For this review, take the finished solid that the model builds, in its own axes (mm). Face numbers are marked on the shaded views. Coordinates: 2 decimals unless noted, no trailing zeros. Write each loop counter-clockwise with the first axis right and the second up, starting at its lowest first coordinate (ties: lowest second). Pieces come first, ordered by that corner, then holes. Notation, with made-up numbers: (-20, 86) - (-8, 86) arc R23 ccw to (-8, 125) - close; hole circle Ø1 at (56.25, 42). An arc over 180 degrees is marked (long way). Use one line per item in the form item = value. Start each with the question number.
1) Insertion check: P1, Ø10, axis at x = -2.5, y = -7.5, coming from the +Z side; P2, Ø6, axis at y = 20, z = 50.5, coming from the +X side; P3, Ø5, axis at x = -4, z = 50, coming from the -Y side; P4, Ø6, axis at y = -4, z = 32, coming from the +X side. Each pin has a flat end and moves straight along its axis. Give the tip position at first contact, or say it passes through.
2) Mouldability with a two-part tool opening along X and no side actions: class the marked faces 1, 2, 3 and 4 as pulls with the +X half, pulls with the -X half, needs draft (parallel to the pull), parting line crosses it, or undercut.
3) We need section B-B (x = -0.5). Give the boundary of the cut face in (y, z).
4) We need section C-C (y = 40). Give the boundary of the cut face in (x, z).
5) We need section A-A (z = 37). Give the boundary of the cut face in (x, y), plus the area to 3 significant figures.
6) For L1, parallel to X at y = 24, z = 19; L2, parallel to X at y = -11, z = 22; L3, parallel to Y at x = -20, z = 57, list the stretches that pass through material, from the lowest coordinate up. Write a range as from..to.
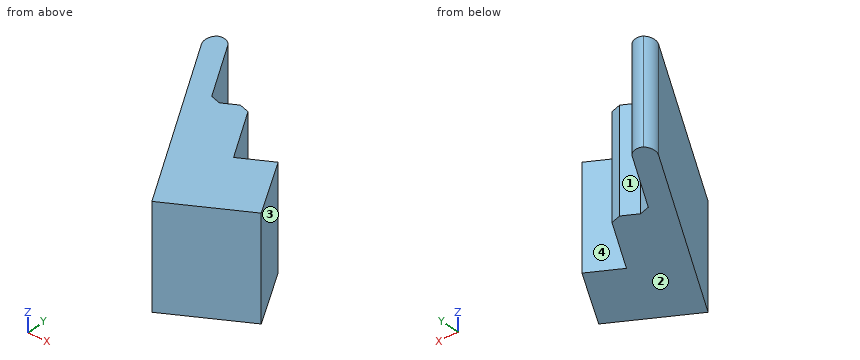
```python
from build123d import *

# Parameters (mm, degrees)
F1_DEPTH    = 72.644
F2_R        = 7.3585229381
F3_SIZE     = 5.08
F4_SIZE     = 5.08
F5_T1_DEPTH = 116.8137644874


# Not quite as in the source:
# - a fillet or chamfer that OpenCascade refuses, or shapes differently, is made with other operations: its cross-section is extruded or revolved along the edge and cut away or added


with BuildPart() as f1:
    # F0 (on Top) → F1 (new body)
    with BuildSketch(Plane.XY):
        Polygon((-24.6386431996, 69.7602594984), (-36.737293005, 62.7278536558), (40.861338377, -70.7739219069), (91.9838476343, -41.0586860274), (68.6385333538, 0), (47.8052062724, -12.1094844007), (23.9140867359, 28.9931332809), (5.3346716929, 18.1937474815), align=None)
    extrude(amount=F1_DEPTH)

    # F2
    f2_edges = [f1.edges().sort_by_distance(p)[0] for p in [
        (-24.638643, 69.760259, 36.322),
    ]]
    fillet(f2_edges, radius=F2_R)

    # F3
    f3_edges = [f1.edges().sort_by_distance(p)[0] for p in [
        (5.334672, 18.193747, 36.322),
    ]]
    chamfer(f3_edges, length=F3_SIZE)

    # F4
    f4_edges = [f1.edges().sort_by_distance(p)[0] for p in [
        (23.914087, 28.993133, 36.322),
    ]]
    chamfer(f4_edges, length=F4_SIZE)

    # F5: fillet of radius 9.1981536726 on 1 edges, made by hand

    # F5_s2 → F5_t1 (cut)
    with BuildSketch(Plane.XY.offset(-22.0848822437)):
        with BuildLine():
            ThreePointArc((-31.0005259261, 66.0623806462), (-33.480123973, 60.7928785055), (-32.2979662711, 55.0903735776))
            Line((-32.2979662711, 55.0903735776), (-36.737293005, 62.7278536558))
            Line((-36.737293005, 62.7278536558), (-31.0005259261, 66.0623806462))
        make_face()
    extrude(amount=F5_T1_DEPTH, mode=Mode.SUBTRACT)


solid = f1.part
```
Determined:
q1.P1 = through
q1.P2 = 30.89
q1.P3 = 2.11
q1.P4 = 72.62
q2.face_1 = undercut
q2.face_2 = needs draft
q2.face_3 = pulls with the +X half
q2.face_4 = undercut
q3.outline = (0.38, 0) - (28.23, 0) - (28.23, 72.64) - (0.38, 72.64) - close
q4.outline = (-23.53, 0) - (-7.34, 0) - (-7.34, 72.64) - (-23.53, 72.64) - close
q5.outline = (-32.3, 55.09) - (40.86, -70.77) - (91.98, -41.06) - (68.64, 0) - (47.81, -12.11) - (26.47, 24.6) - (19.52, 26.44) - (9.73, 20.75) - (2.78, 22.59) - (-20.94, 63.4) arc R7.36 ccw to (-31, 66.06) arc R9.2 ccw to start
q5.area = 5,300 mm²
q6.L1 = -14.23..1.96, 15.32..26.82
q6.L2 = 6.12..47.16, 49.71..74.89
q6.L3 = 33.93..61.78
